Source: CAD feature listing. Evaluate the final solid. Frame: model axes, mm. Coordinates: 2 decimals unless noted, no trailing zeros. Loops run counter-clockwise (first coordinate to the right, second up) from the corner with the lowest first, then second, coordinate; pieces in that order, holes last.
Item 1: Pin query (flat end, axial travel): pin 1 Ø12 at (y, z) = (16.5, -14.5) entering from -X; pin 2 Ø6 at (x, z) = (4, 7.5) entering from -Y; pin 3 Ø6 at (x, y) = (-5.5, -7.5) entering from +Z. Return the tip coordinate at first contact, or that it passes through.
Item 2: Section query A-A, the plane x = -13.5. Return the cut outline in (y, z), then the cut area to 3 significant figures.
Item 3: Section query B-B, the plane z = -4.5. Return the cut outline in (x, y).
Item 4: Section query C-C, the plane y = 4. Return the cut outline in (x, z).
Item 5: Section query D-D, the plane x = -7. Return the cut outline in (y, z) (3 decimals), then the cut area to 3 significant figures.
Item 6: Line query: probe 1 along X at (y, z) = (2.5, -8); probe 2 along X at (y, z) = (-5, 1); probe 3 along Z at (x, y) = (-9, -7.5). Output: solid intervals per line, ascending.
```python
from build123d import *

# Parameters (mm, degrees)
F1_ANGLE = -180
F3_ANGLE = 250


with BuildPart() as f1:
    # F0 (on Front) → F1 (revolve)
    with BuildSketch(Plane.XZ):
        with BuildLine():
            Line((0, -20), (0, -21))
            ThreePointArc((0, -21), (21, 0), (0, 21))
            Line((0, 21), (0, 20))
            ThreePointArc((0, 20), (20, 0), (0, -20))
        make_face()
    revolve(axis=Axis((0, 0, 0), (0, 0, -1)), revolution_arc=F1_ANGLE)

    # F2 (on Front) → F3 (revolve)
    with BuildSketch(Plane.XZ):
        with BuildLine():
            Line((10, 0), (20, 0))
            ThreePointArc((20, 0), (0, 20), (-20, 0))
            Line((-20, 0), (-10, 0))
            ThreePointArc((-10, 0), (0, 10), (10, 0))
        make_face()
    revolve(axis=Axis((0, 0, 0), (-1, 0, 0)), revolution_arc=F3_ANGLE)

    # F4 (on Front) → F5 (revolve)
    with BuildSketch(Plane.XZ):
        with BuildLine():
            Line((10, 0), (-10, 0))
            ThreePointArc((-10, 0), (0, -10), (10, 0))
        make_face()
    revolve(axis=Axis((0, 0, 0), (1, 0, 0)))


solid = f1.part
```
Verdict:
1. pin 1: stops at x = -13.64
1. pin 2: stops at y = -8.35
1. pin 3: stops at z = 7.77
2. outline: (-13.87, -5.05) arc R14.76 ccw to (0, -14.76) - (0, -16.09) arc R16.09 ccw to (0, 16.09) - (0, 0) - close
2. area: 539 mm2
3. outline: (-20.51, 0) - (-19.49, 0) arc R19.49 ccw to (-15.06, -12.36) - (15.06, -12.36) arc R19.49 ccw to (19.49, 0) - (20.51, 0) arc R20.51 ccw to start
4. outline: circle Ø41.23 at (0, 0)
5. outline: (-17.605, -6.408) arc R18.735 ccw to (0, -18.735) - (0, -19.799) arc R19.799 ccw to (0, 19.799) - (0, 7.141) arc R7.141 ccw to (-6.711, -2.443) - close
5. area: 879 mm2
6. probe 1: x = -19.25 to 19.25
6. probe 2: x = -8.6 to 8.6
6. probe 3: z = -16.21 to -2.73
